Answer from the drawing. Dimensions are ordinates in mm from the lowest x, y and z of the part. Give positions to 0.01 mm unless a question says otherwise; leave off trailing zeros. Loops run counter-clockwise (first coordinate to the right, second up) from the corner with the lowest first, then second, coordinate; pieces in that order, holes last.
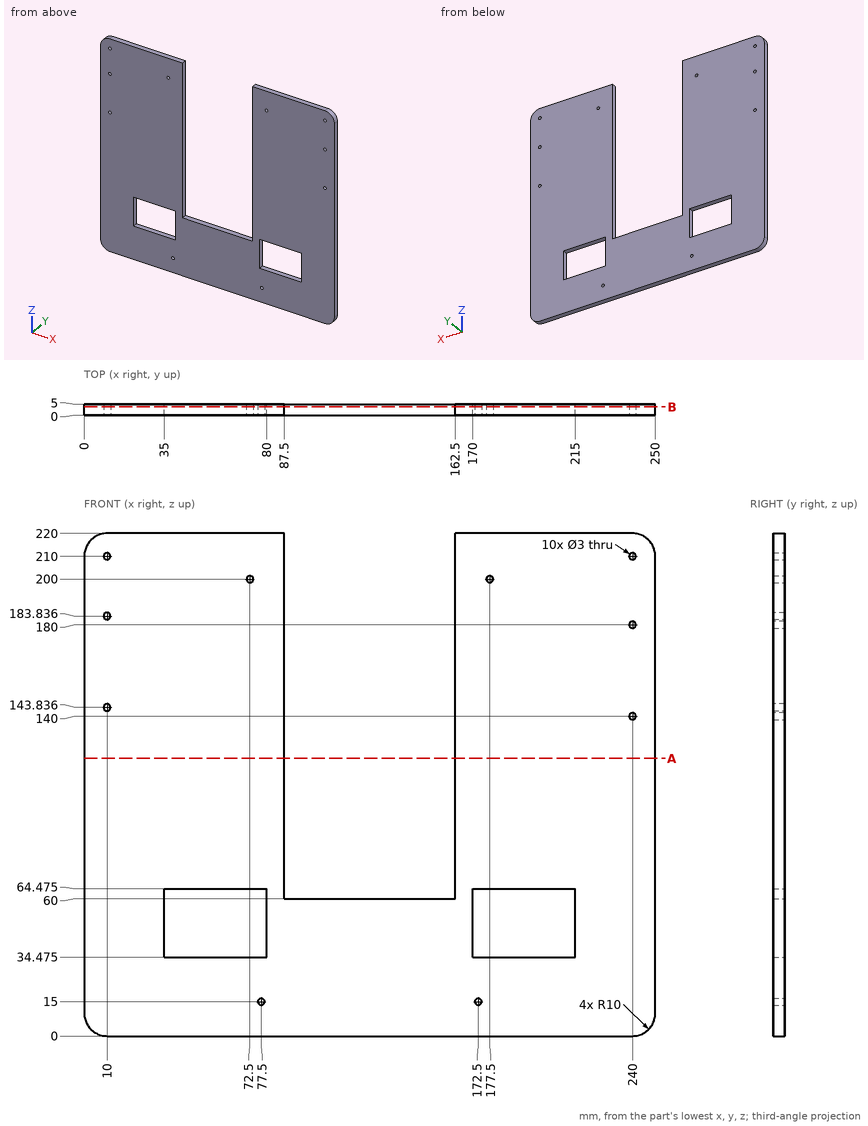
Item 1: Consider line 1 (Z direction, x = 77.5, y = 1.45) (1 decimal); line 2 (X direction, y = 1.95, z = 140); line 3 (Z direction, x = 72.5, y = 1.55) (1 decimal). Determine where each line is inside the solid, lowest interval first.
Item 2: Find section B-B, the plane y = 3.7. Give the number of separate pieces and of enclosed holes in the cut face, plus the area to 3 significant figures.
Item 3: Find section A-A, the plane z = 121.5. Write down the section's boundary in (x, y), plus the area to 3 significant figures.
Ans:
1. line 1: z = 0 to 13.5, 16.5 to 34.5, 64.5 to 220
1. line 2: x = 0 to 87.5, 162.5 to 238.5, 241.5 to 250
1. line 3: z = 0 to 34.5, 64.5 to 198.5, 201.5 to 220
2. separate pieces: 1
2. enclosed holes: 12
2. area: 40,100 mm2
3. outline: (0, 0) - (87.5, 0) - (87.5, 5) - (0, 5) - close; (162.5, 0) - (250, 0) - (250, 5) - (162.5, 5) - close
3. area: 875 mm2
